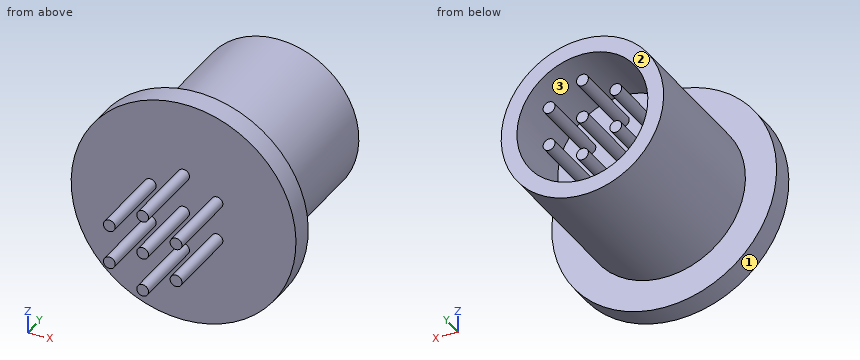
from build123d import *

# Parameters (mm, degrees)
SKETCH1_R           = 10.3
BOSS_EXTRUDE1_DEPTH = 20
SKETCH2_R           = 14.25
BOSS_EXTRUDE2_DEPTH = 3
SKETCH3_R           = 8.3
CUT_EXTRUDE1_DEPTH  = 10
SKETCH4_R           = 0.75
BOSS_EXTRUDE3_DEPTH = 10
BOSS_EXTRUDE4_START = 10
SKETCH5_R           = 0.75
BOSS_EXTRUDE4_DEPTH = 10


with BuildPart() as part:
    # Sketch1 → Boss-Extrude1 (new body)
    with BuildSketch(Plane(origin=(0, 0, 0), x_dir=(1, 0, 0), z_dir=(0, 1, 0))):
        with Locations(Location((0, 0, 0), (0, 0, 270))):
            Circle(SKETCH1_R)
    extrude(amount=BOSS_EXTRUDE1_DEPTH)

    # Sketch2 → Boss-Extrude2 (add)
    with BuildSketch(Plane.XZ):
        with Locations(Location((0, 0, 0), (0, 0, 270))):
            Circle(SKETCH2_R)
    extrude(amount=BOSS_EXTRUDE2_DEPTH)

    # Sketch3 → Cut-Extrude1 (cut)
    with BuildSketch(Plane(origin=(0, 20, 0), x_dir=(1, 0, 0), z_dir=(0, 1, 0))):
        with Locations(Location((0, 0, 0), (0, 0, 270))):
            Circle(SKETCH3_R)
    extrude(amount=-CUT_EXTRUDE1_DEPTH, mode=Mode.SUBTRACT)

    # Sketch4 → Boss-Extrude3 (add)
    with BuildSketch(Plane(origin=(0, 10, 0), x_dir=(1, 0, 0), z_dir=(0, 1, 0))):
        with Locations(Location((0, 4.884385532, 0), (0, 0, 270))):
            Circle(SKETCH4_R)
        with Locations(Location((4.230001953, 2.442192766, 0), (0, 0, 270))):
            Circle(SKETCH4_R)
        with Locations(Location((4.230001953, -2.442192766, 0), (0, 0, 270))):
            Circle(SKETCH4_R)
        with Locations(Location((0, -4.884385532, 0), (0, 0, 270))):
            Circle(SKETCH4_R)
        with Locations(Location((-4.230001953, -2.442192766, 0), (0, 0, 270))):
            Circle(SKETCH4_R)
        with Locations(Location((-4.230001953, 2.442192766, 0), (0, 0, 270))):
            Circle(SKETCH4_R)
        with Locations(Location((0, 0, 0), (0, 0, 270))):
            Circle(SKETCH4_R)
    extrude(amount=BOSS_EXTRUDE3_DEPTH)

    # Sketch5 → Boss-Extrude4 (add)
    with BuildSketch(Plane.XZ.offset(3).offset(BOSS_EXTRUDE4_START)):
        with Locations(Location((0, 0, 0), (0, 0, 90))):
            Circle(SKETCH5_R)
        with Locations(Location((-4.230001953, -2.442192766, 0), (0, 0, 90))):
            Circle(SKETCH5_R)
        with Locations(Location((-4.230001953, 2.442192766, 0), (0, 0, 90))):
            Circle(SKETCH5_R)
        with Locations(Location((0, 4.884385532, 0), (0, 0, 90))):
            Circle(SKETCH5_R)
        with Locations(Location((4.230001953, 2.442192766, 0), (0, 0, 90))):
            Circle(SKETCH5_R)
        with Locations(Location((4.230001953, -2.442192766, 0), (0, 0, 90))):
            Circle(SKETCH5_R)
        with Locations(Location((0, -4.884385532, 0), (0, 0, 90))):
            Circle(SKETCH5_R)
    extrude(amount=-BOSS_EXTRUDE4_DEPTH)


solid = part.part
Geometry: final body of the model. Coordinates: model frame, mm. Face numbers are marked on the shaded views. Round coordinates to 2 decimals unless told otherwise and drop trailing zeros. Order: outer loops, then holes, each group sorted by start corner. A loop starts at its lowest first (then second) coordinate and runs counter-clockwise, first axis right, second up. Notation, with made-up numbers: (72, -33) -> (104, -33) arc R20 cw to (104, 5) -> close; hole circle Ø6 at (70.5, 49). An arc over 180 degrees is marked (long way). Put each result on its own line as item: value. Start each with the question number.
Q1. Line query: probe 1 along X at (y, z) = (12.75, 0); probe 2 along Y at (x, z) = (7.75, -5.75); probe 3 along Y at (x, z) = (-10.75, -0.5). Output: solid intervals per line, ascending.
Q2. Section D-D on x = 1.75. Return the cut outline in (y, z), and give its area (3 significant figures).
Q3. Section B-B on y = -9. Return the cut outline in (x, z), and give its area (3 significant figures).
Q4. Section C-C on z = 9. Return the cut outline in (x, y), and give its area (3 significant figures).
Q5. First-contact query: pin 1 (4 mm diameter, centred on x = 4, z = 9, fed in from -Y); pin 2 (3 mm diameter, centred on y = -9, z = -2.5, fed in from -X); pin 3 (3 mm diameter, centred on x = 3.5, y = 16.5, fed in from +Z). Flat tips, straight axial feed; report the tip coordinate or a pass-through.
Q6. Pull-direction query (X, two-part tool) for the marked faces 1, 2 and 3; classes: +X half, -X half, draft (parallel to the pull), parting line (faces both ways), or undercut.
Q7. Section A-A on y = 16.5. Give the number of separate pieces and of enclosed holes in the cut face, and give its area (3 significant figures).
Ans:
1. probe 1: x = -10.3 to -8.3, -0.75 to 0.75, 8.3 to 10.3
1. probe 2: y = -3 to 20
1. probe 3: y = -3 to 0
2. outline: (-3, -14.14) -> (0, -14.14) -> (0, -10.15) -> (20, -10.15) -> (20, -8.11) -> (10, -8.11) -> (10, 8.11) -> (20, 8.11) -> (20, 10.15) -> (0, 10.15) -> (0, 14.14) -> (-3, 14.14) -> close
2. area: 329 mm2
3. outline: circle Ø1.5 at (-4.23, -2.44); circle Ø1.5 at (-4.23, 2.44); circle Ø1.5 at (0, -4.88); circle Ø1.5 at (0, 0); circle Ø1.5 at (0, 4.88); circle Ø1.5 at (4.23, -2.44); circle Ø1.5 at (4.23, 2.44)
3. area: 12.4 mm2
4. outline: (-11.05, -3) -> (11.05, -3) -> (11.05, 0) -> (5.01, 0) -> (5.01, 20) -> (-5.01, 20) -> (-5.01, 0) -> (-11.05, 0) -> close
4. area: 267 mm2
5. pin 1: stops at y = -3
5. pin 2: stops at x = -4.98
5. pin 3: stops at z = 10.1
6. face 1: parting line
6. face 2: draft
6. face 3: undercut
7. separate pieces: 8
7. enclosed holes: 1
7. area: 129 mm2
